```python
from build123d import *

# Parameters (mm, degrees)
SKETCH1_W           = 48.7
SKETCH1_H           = 26
SKETCH1_R           = 1.5
BOSS_EXTRUDE1_DEPTH = 1.65
SKETCH2_W           = 38.5
SKETCH2_H           = 3
BOSS_EXTRUDE2_DEPTH = 11.3
SKETCH3_W           = 80
SKETCH3_H           = 20
BOSS_EXTRUDE3_DEPTH = 5


with BuildPart() as part:
    # Sketch1 → Boss-Extrude1 (new body)
    with BuildSketch(Plane(origin=(0, 0, 0), x_dir=(1, 0, 0), z_dir=(0, 1, 0))):
        Rectangle(SKETCH1_W, SKETCH1_H)
        with Locations(Location((-21.95, 10.6, 0), (0, 0, 270))):
            Circle(SKETCH1_R, mode=Mode.SUBTRACT)
        with Locations(Location((-21.95, -10.6, 0), (0, 0, 90))):
            Circle(SKETCH1_R, mode=Mode.SUBTRACT)
        with Locations(Location((21.95, -10.6, 0), (0, 0, 270))):
            Circle(SKETCH1_R, mode=Mode.SUBTRACT)
        with Locations(Location((21.95, 10.6, 0), (0, 0, 90))):
            Circle(SKETCH1_R, mode=Mode.SUBTRACT)
    extrude(amount=BOSS_EXTRUDE1_DEPTH)

    # Sketch2 → Boss-Extrude2 (add)
    with BuildSketch(Plane(origin=(0, 1.65, 0), x_dir=(1, 0, 0), z_dir=(0, 1, 0))):
        with Locations((0.2, 11.5)):
            Rectangle(SKETCH2_W, SKETCH2_H)
        with Locations((0.2, -11.5)):
            Rectangle(SKETCH2_W, SKETCH2_H)
    extrude(amount=BOSS_EXTRUDE2_DEPTH)

    # Sketch3 → Boss-Extrude3 (add)
    with BuildSketch(Plane(origin=(0, 1.65, 0), x_dir=(1, 0, 0), z_dir=(0, 1, 0))):
        with Locations((-24.35, 0)):
            Rectangle(SKETCH3_W, SKETCH3_H)
    extrude(amount=BOSS_EXTRUDE3_DEPTH)


solid = part.part
```
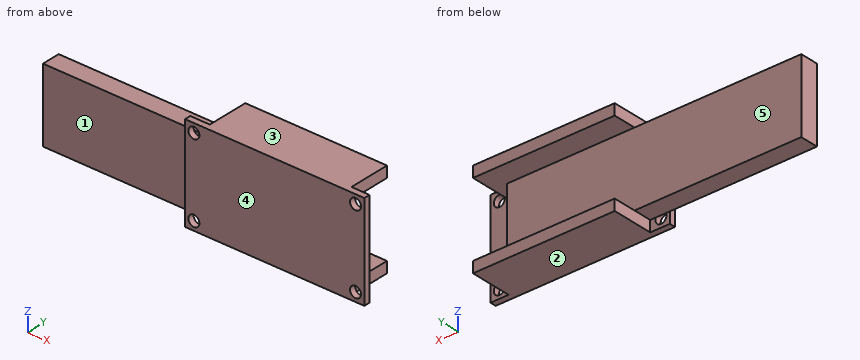
The model under review builds one solid part; all positions refer to its coordinate system, in mm. Face numbers are marked on the shaded views. A direction names the side the tool comes from. Coordinates: 2 decimals unless noted, no trailing zeros. Write each loop counter-clockwise with the first axis right and the second up, starting at its lowest first coordinate (ties: lowest second). Pieces come first, ordered by that corner, then holes.
1) Machinability: for the marked faces 1 and 2, which of the approach directions +Z, -Z, +X, -X, +Y, -Y give a long, thin tool a straight path to every point of the face, cutting with its end or side? Answer none if there is none.
2) We need section A-A on y = 10. State the section outline as (x, z) points.
3) Clearance check with flat-ended pins moving along their axes: pin 1 Ø2.5 at (x, z) = (-21.95, 10.6) entering from +Y; pin 2 Ø0.9 at (y, z) = (7.5, 12) entering from -X; pin 3 Ø1.5 at (y, z) = (7.5, 12) entering from +X. State where each tip first meets the part, or that it passes through.
4) We need section D-D on y = 3.25. State the section outline as (x, z) points, then the cut area to 3 significant figures.
5) The part is to be moulded in two halves that separate along Z. For the marked faces 3, 4 and 5, say which applies: pulls with the +Z half, pulls with the -Z half, needs draft (parallel to the pull), parting line crosses it, or undercut.
6) To check wall thickness, follow probe 1 along Z at (x, y) = (-21.95, 0.9); probe 2 along X at (y, z) = (0.8, -10.6); probe 3 along Z at (x, y) = (-31, 1.75). State the ranges of each line that lie inside material, in increasing order.
7) We need section C-C on z = -4. State the section outline as (x, y) points.
8) We need section B-B on x = -21.95. State the section outline as (y, z) points.
Answer list:
1. face 1: +Z, -Z, -X, -Y
1. face 2: -Z, +X, -X, +Y, -Y
2. outline: (-19.05, -13) - (19.45, -13) - (19.45, -10) - (-19.05, -10) - close; (-19.05, 10) - (19.45, 10) - (19.45, 13) - (-19.05, 13) - close
3. pin 1: stops at y = 6.65
3. pin 2: stops at x = -19.05
3. pin 3: stops at x = 19.45
4. outline: (-64.35, -10) - (-19.05, -10) - (-19.05, -13) - (19.45, -13) - (19.45, -10) - (15.65, -10) - (15.65, 10) - (19.45, 10) - (19.45, 13) - (-19.05, 13) - (-19.05, 10) - (-64.35, 10) - close
4. area: 1,830 mm2
5. face 3: pulls with the +Z half
5. face 4: needs draft
5. face 5: undercut
6. probe 1: z = -13 to -12.1, -9.1 to 9.1, 12.1 to 13
6. probe 2: x = -24.35 to -23.45, -20.45 to 20.45, 23.45 to 24.35
6. probe 3: z = -10 to 10
7. outline: (-64.35, 1.65) - (-24.35, 1.65) - (-24.35, 0) - (24.35, 0) - (24.35, 1.65) - (15.65, 1.65) - (15.65, 6.65) - (-64.35, 6.65) - close
8. outline: (0, -13) - (1.65, -13) - (1.65, -12.1) - (0, -12.1) - close; (0, -9.1) - (1.65, -9.1) - (1.65, -10) - (6.65, -10) - (6.65, 10) - (1.65, 10) - (1.65, 9.1) - (0, 9.1) - close; (0, 12.1) - (1.65, 12.1) - (1.65, 13) - (0, 13) - close
